Check sheet for the modelled part. Datum: model origin and axes. Units: mm. Face numbers are marked on the shaded views. Coordinates: 2 decimals unless noted, no trailing zeros. Loops run counter-clockwise (first coordinate to the right, second up) from the corner with the lowest first, then second, coordinate; pieces in that order, holes last.
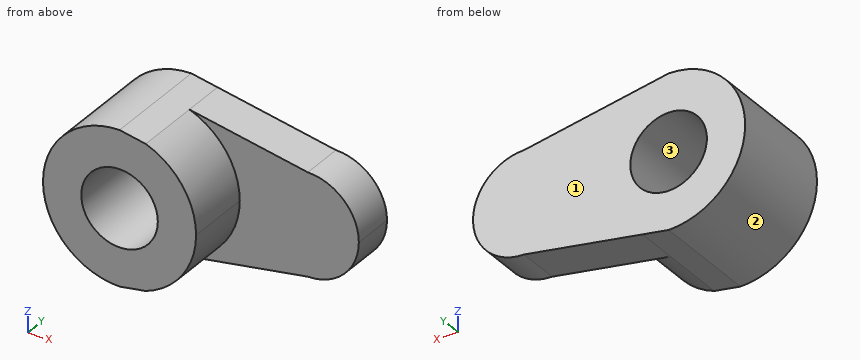
```python
from build123d import *

# Parameters (mm, degrees)
F0_R     = 14.2875
F1_DEPTH = 40.2336
F2_DEPTH = 15.7734


with BuildPart() as f1:
    # F0 (on Front) → F1 (new body)
    with BuildSketch(Plane.XZ):
        with BuildLine():
            ThreePointArc((-44.194295302, -26.8489932886), (-30.5654478712, -16.3866864902), (-25.4, 0))
            ThreePointArc((-25.4, 0), (-30.5654478712, 16.3866864902), (-44.194295302, 26.8489932886))
            Line((-44.194295302, 26.8489932886), (-53.975, 28.575))
            ThreePointArc((-53.975, 28.575), (-82.55, 0), (-53.975, -28.575))
            Line((-53.975, -28.575), (-44.194295302, -26.8489932886))
        make_face()
        with Locations((-53.975, 0)):
            Circle(F0_R, mode=Mode.SUBTRACT)
    extrude(amount=F1_DEPTH)

    # F0 (on Front) → F2 (join)
    with BuildSketch(Plane.XZ):
        with BuildLine():
            ThreePointArc((0, 19.05), (-13.4703841816, 13.4703841816), (-19.05, 0))
            ThreePointArc((-19.05, 0), (-13.4703841816, -13.4703841816), (0, -19.05))
            ThreePointArc((0, -19.05), (13.4703841816, -13.4703841816), (19.05, 0))
            ThreePointArc((19.05, 0), (13.4703841816, 13.4703841816), (0, 19.05))
        make_face()
        with BuildLine():
            ThreePointArc((-10.16, 0), (0, 10.16), (10.16, 0))
            ThreePointArc((10.16, 0), (0, -10.16), (-10.16, 0))
        make_face(mode=Mode.SUBTRACT)
        with BuildLine():
            Line((-25.4, 0), (-19.05, 0))
            ThreePointArc((-19.05, 0), (-13.4703841816, 13.4703841816), (0, 19.05))
            Line((0, 19.05), (-44.194295302, 26.8489932886))
            ThreePointArc((-44.194295302, 26.8489932886), (-30.5654478712, 16.3866864902), (-25.4, 0))
        make_face()
        with BuildLine():
            ThreePointArc((0, -19.05), (-13.4703841816, -13.4703841816), (-19.05, 0))
            Line((-19.05, 0), (-25.4, 0))
            ThreePointArc((-25.4, 0), (-30.5654478712, -16.3866864902), (-44.194295302, -26.8489932886))
            Line((-44.194295302, -26.8489932886), (0, -19.05))
        make_face()
        with BuildLine():
            ThreePointArc((-10.16, 0), (0, -10.16), (10.16, 0))
            ThreePointArc((10.16, 0), (0, 10.16), (-10.16, 0))
        make_face()
    extrude(amount=F2_DEPTH)


solid = f1.part
```
1) Section check A-A on z = -7. Enter the section's corners in (x, y), plus the area to 3 significant figures.
Answer sheet:
outline: (-81.68, -40.23) - (-66.43, -40.23) - (-66.43, 0) - (-81.68, 0) - close; (-41.52, -40.23) - (-26.27, -40.23) - (-26.27, -15.77) - (17.72, -15.77) - (17.72, 0) - (-41.52, 0) - close
area: 1,920 mm2
2) Section check C-C on x = -58.5. Enter the section's corners in (y, z).
Answer sheet:
outline: (-40.23, -28.21) - (0, -28.21) - (0, -13.55) - (-40.23, -13.55) - close; (-40.23, 13.55) - (0, 13.55) - (0, 28.21) - (-40.23, 28.21) - close
3) Depth check by flat-ended pin: pin 1 (1 mm diameter, centred on y = -11, z = -9, fed in from +X); pin 2 (8 mm diameter, centred on x = -46.5, z = 1.5, fed in from -Y); pin 3 (10 mm diameter, centred on y = -5, z = -20, fed in from -X); pin 4 (4 mm diameter, centred on y = -22, z = 7.5, fed in from -X). Enter the tip coordinate at first touch or a pass-through.
Answer sheet:
pin 1: stops at x = 17.05
pin 2: passes through
pin 3: stops at x = -78.3
pin 4: stops at x = -82.02
4) Scan lines: line 1 (X direction, y = -5, z = 0.5); line 2 (Z direction, x = -50, y = -36.5); line 3 (X direction, y = -8, z = -13). Record each from-to range of solid material in increasing order.
Answer sheet:
line 1: x = -82.55 to -68.25, -39.7 to 19.04
line 2: z = -27.87 to -13.72, 13.72 to 27.87
line 3: x = -79.42 to -59.9, -48.05 to 13.92
5) Section check D-D on z = 9. Enter the section's corners in (x, y).
Answer sheet:
outline: (-81.1, -40.23) - (-65.07, -40.23) - (-65.07, 0) - (-81.1, 0) - close; (-42.88, -40.23) - (-26.85, -40.23) - (-26.85, -15.77) - (16.79, -15.77) - (16.79, 0) - (-42.88, 0) - close
6) Mould release check, pull along X, two halves, no side actions. Record for the marked faces 1, 2 and 3: +X half, -X half, draft (parallel to the pull), parting line (faces both ways), or undercut.
Answer sheet:
face 1: draft
face 2: -X half
face 3: undercut
